Here's how the part is built. I have some questions about the finished solid (model axes, mm). A direction names the side the tool comes from. Coordinates: 2 decimals unless noted, no trailing zeros. Write each loop counter-clockwise with the first axis right and the second up, starting at its lowest first coordinate (ties: lowest second). Pieces come first, ordered by that corner, then holes.
Item 1: I'm going to push flat-ended pins straight in: pin 1 Ø2 at (y, z) = (0, -37) entering from -X; pin 2 Ø6 at (x, y) = (-19.5, -4) entering from -Z; pin 3 Ø2.5 at (x, z) = (6.15, -18) entering from +Y; pin 4 Ø1.6 at (x, z) = (-6, -39) entering from -Y. Where does each tip first touch, or does it pass through?
Item 2: If we section it at A-A (z = 0): Please give me the cut outline in (x, y), then the cut area to 3 significant figures.
Item 3: For faces 1 (the face through (0.42, 8.898, 57.285)), 2 (the face through (-0.66, -17.662, 14.985)), which set-ups out of +Z, -Z, +X, -X, +Y, -Y let a thin tool reach every point of the face, with its end or its side?
Item 4: If we section it at C-C (x = 18.5): Please give me the cut outline in (y, z).
Item 5: If we section it at B-B (y = 0): Please give me the cut outline in (x, z).
Item 6: If we section it at D-D (y = -20): Please give me the cut outline in (x, z).
Item 7: We'd pull the mould along Y, two halves only. Please class faces 3 (the face through (0, 0, -54)), 4 (the face through (30, -2, 1)), 5 (the face through (14, -11.5, 12)): +Y half, -Y half, draft (parallel to the pull), parting line (faces both ways), or undercut.
Item 8: If I drill on line 1 (X direction, y = -5, z = -39); line 2 (Z direction, x = -18, y = 3); line 3 (Z direction, x = 19.5, y = -2.5), over which ranges is the centre line in solid material (lowest first)?
from build123d import *

# Parameters (mm, degrees)
SKETCH1_R           = 7.5
SKETCH1_R_2         = 4
BOSS_EXTRUDE1_DEPTH = 30
SKETCH2_W           = 15
SKETCH2_H           = 12.5
SKETCH3_R           = 10
CUT_EXTRUDE1_DEPTH  = 73.031243221
SKETCH4_R           = 1.05
CUT_EXTRUDE2_DEPTH  = 10


with BuildPart() as part:
    # Sketch1 → Boss-Extrude1 (new, symmetric)
    with BuildSketch(Plane(origin=(0, 0, 0), x_dir=(0, 0, -1), z_dir=(1, 0, 0))):
        with BuildLine():
            Line((-50, -11.5), (50, -11.5))
            ThreePointArc((50, -11.5), (57.582875444, 8.645808233), (38.598245749, -1.5))
            Line((38.598245749, -1.5), (-38.598245749, -1.5))
            ThreePointArc((-38.598245749, -1.5), (-57.582875444, 8.645808233), (-50, -11.5))
        make_face()
        with Locations(Location((-50, 0, 0), (0, 0, 180))):
            Circle(SKETCH1_R, mode=Mode.SUBTRACT)
        with Locations(Location((50, 0, 0), (0, 0, 180))):
            Circle(SKETCH1_R_2, mode=Mode.SUBTRACT)
    extrude(amount=BOSS_EXTRUDE1_DEPTH, both=True)

    # Sketch2 → Revolve1 (revolve)
    with BuildSketch(Plane(origin=(0, 0, 0), x_dir=(0, 0, -1), z_dir=(1, 0, 0))):
        with Locations((7.5, -17.75)):
            Rectangle(SKETCH2_W, SKETCH2_H)
    revolve(axis=Axis((0, -24, 0), (0, 1, 0)))

    # Sketch3 → Cut-Extrude1 (cut, through all)
    with BuildSketch(Plane(origin=(0, -1.5, 0), x_dir=(1, 0, 0), z_dir=(0, 1, 0))):
        with Locations(Location((0, 0, 0), (0, 0, 270))):
            Circle(SKETCH3_R)
    extrude(amount=-CUT_EXTRUDE1_DEPTH, mode=Mode.SUBTRACT)

    # Sketch4 → Cut-Extrude2 (cut)
    with BuildSketch(Plane.XZ.offset(11.5)):
        with Locations(Location((-6.15, -18, 0), (0, 0, 270))):
            Circle(SKETCH4_R)
        with Locations(Location((-6.15, -39, 0), (0, 0, 270))):
            Circle(SKETCH4_R)
        with Locations(Location((6.15, -18, 0), (0, 0, 270))):
            Circle(SKETCH4_R)
        with Locations(Location((6.15, -39, 0), (0, 0, 270))):
            Circle(SKETCH4_R)
    extrude(amount=-CUT_EXTRUDE2_DEPTH, mode=Mode.SUBTRACT)


solid = part.part
Answer list:
1. pin 1: passes through
1. pin 2: stops at z = -61.46
1. pin 3: stops at y = -1.5
1. pin 4: stops at y = -1.5
2. outline: (-30, -11.5) - (-15, -11.5) - (-15, -24) - (-10, -24) - (-10, -1.5) - (-30, -1.5) - close; (10, -24) - (15, -24) - (15, -11.5) - (30, -11.5) - (30, -1.5) - (10, -1.5) - close
2. area: 525 mm2
3. face 1: +X, -X
3. face 2: -Y
4. outline: (-11.5, -50) arc R11.5 ccw (long way) to (-1.5, -38.6) - (-1.5, 38.6) arc R11.5 ccw (long way) to (-11.5, 50) - close; hole circle Ø15 at (0, 50); hole circle Ø8 at (0, -50)
5. outline: (-30, -61.5) - (30, -61.5) - (30, -54) - (-30, -54) - close; (-30, -46) - (30, -46) - (30, -38.5) - (-30, -38.5) - close; (-30, 38.5) - (30, 38.5) - (30, 42.5) - (-30, 42.5) - close; (-30, 57.5) - (30, 57.5) - (30, 61.5) - (-30, 61.5) - close
6. outline: circle Ø30 at (0, 0); hole circle Ø20 at (0, 0)
7. face 3: undercut
7. face 4: draft
7. face 5: -Y half
8. line 1: x = -30 to -7.2, -5.1 to 5.1, 7.2 to 30
8. line 2: z = -61.1 to -52.65, -47.35 to -38.9, 38.9 to 43.13, 56.87 to 61.1
8. line 3: z = -61.22 to -53.12, -46.88 to 42.93, 57.07 to 61.22
